```python
from build123d import *

# Parameters (mm, degrees)
BOSS_EXTRUDE1_DEPTH      = 10
BOSS_EXTRUDE2_DEPTH      = 15
BOSS_EXTRUDE2_DEPTH_BACK = 5
SKETCH1_3_R              = 3
SKETCH2_R                = 1.5
CUT_EXTRUDE1_DEPTH       = 39.79576151
BOSS_EXTRUDE3_DEPTH      = 5
BOSS_EXTRUDE3_DEPTH_BACK = 15
SKETCH3_R                = 3


with BuildPart() as part:
    # Sketch1 → Boss-Extrude1 (new body)
    with BuildSketch(Plane.XY):
        with BuildLine():
            Line((-20, 10), (-20, -10))
            Line((-20, -10), (-2.846049894, -15.717983369))
            ThreePointArc((-2.846049894, -15.717983369), (0, -13.666666667), (2.846049894, -15.717983369))
            Line((2.846049894, -15.717983369), (20, -10))
            Line((20, -10), (20, 10))
            Line((20, 10), (-20, 10))
        make_face()
    extrude(amount=BOSS_EXTRUDE1_DEPTH)

    # Sketch1_3 → Boss-Extrude2 (add, two sides: drawn at the far end of the back side and taken through both)
    with BuildSketch(Plane.XY.offset(-BOSS_EXTRUDE2_DEPTH_BACK)):
        with Locations((0, -16.666666667)):
            Circle(SKETCH1_3_R)
    extrude(amount=BOSS_EXTRUDE2_DEPTH + BOSS_EXTRUDE2_DEPTH_BACK)

    # Sketch2 → Cut-Extrude1 (cut, through all)
    with BuildSketch(Plane(origin=(0, 10, 0), x_dir=(1, 0, 0), z_dir=(0, 1, 0))):
        with Locations(Location((-14, -5, 0), (0, 0, 270))):
            Circle(SKETCH2_R)
        with Locations((14, -5)):
            Circle(SKETCH2_R)
    extrude(amount=-CUT_EXTRUDE1_DEPTH, mode=Mode.SUBTRACT)

    # Sketch3 → Boss-Extrude3 (add, two sides: drawn at the far end of the back side and taken through both)
    with BuildSketch(Plane.XY.offset(10).offset(-BOSS_EXTRUDE3_DEPTH_BACK)):
        with Locations((0, 10)):
            Circle(SKETCH3_R)
    extrude(amount=BOSS_EXTRUDE3_DEPTH + BOSS_EXTRUDE3_DEPTH_BACK)


solid = part.part
```
The listing builds one solid part. Answer for the finished solid, in the listing's coordinates (mm). A direction names the side the tool comes from. Round coordinates to 2 decimals unless told otherwise and drop trailing zeros. Loops run counter-clockwise (first coordinate to the right, second up) from the corner with the lowest first, then second, coordinate; pieces in that order, holes last.
Q1. Given pin 1 Ø1.5 at (x, y) = (-5, -3.5) entering from -Z; pin 2 Ø8 at (x, z) = (9, 4.5) entering from +Y; pin 3 Ø6 at (x, y) = (-8.5, 3.5) entering from +Z; pin 4 Ø1.8 at (x, z) = (-14, 5) entering from +Y, each flat-ended and moving along its own axis, determine where each tip first touches the part or whether it passes through.
Q2. Which of the six approach directions +Z, -Z, +X, -X, +Y, -Y give full straight-line access (tool end or side, diameter ignored) to faces 1 (the face through (0, -17, 15)), 2 (the face through (-11, 10, 5))?
Q3. Section D-D, the plane x = 0 is taken. Determine the outline of the cut face in (y, z).
Q4. Find the intervals of material crossed by line 1 (X direction, y = -6.75, z = 5); line 2 (Z direction, x = -14, y = -1.25); line 3 (Z direction, x = -5.5, y = -7), in increasing order.
Q5. For a pull along Y with two mould halves and no side action, classify faces 3 (the face through (-20, 0, 5)), 4 (the face through (0, 13, 5)), 5 (the face through (12, 10, 5)) as released by +Y, released by -Y, zero draft, split by the parting line, or undercut.
Q6. Section B-B, the plane z = 5 is taken. Determine the outline of the cut face in (x, y), then the cut area to 3 significant figures.
Q7. Section C-C, the plane y = -1 is taken. Determine the outline of the cut face in (x, z).
Q8. Section A-A, the plane x = 14 is taken. Determine the outline of the cut face in (y, z), then the cut area to 3 significant figures.
Completed:
1. pin 1: stops at z = 0
1. pin 2: stops at y = 10
1. pin 3: stops at z = 10
1. pin 4: passes through
2. face 1: +Z, +X, -X, +Y, -Y
2. face 2: +Z, -Z, -X, +Y
3. outline: (-19.67, -5) - (-13.67, -5) - (-13.67, 0) - (7, 0) - (7, -5) - (13, -5) - (13, 15) - (7, 15) - (7, 10) - (-13.67, 10) - (-13.67, 15) - (-19.67, 15) - close
4. line 1: x = -20 to -15.5, -12.5 to 12.5, 15.5 to 20
4. line 2: z = 0 to 3.5, 6.5 to 10
4. line 3: z = 0 to 10
5. face 3: zero draft
5. face 4: undercut
5. face 5: released by +Y
6. outline: (-20, -10) - (-15.5, -11.5) - (-15.5, 10) - (-20, 10) - close; (-12.5, -12.5) - (-2.85, -15.72) arc R3 ccw (long way) to (2.85, -15.72) - (12.5, -12.5) - (12.5, 10) - (3, 10) arc R3 ccw to (-3, 10) - (-12.5, 10) - close; (15.5, -11.5) - (20, -10) - (20, 10) - (15.5, 10) - close
6. area: 833 mm2
7. outline: (-20, 0) - (20, 0) - (20, 10) - (-20, 10) - close; hole circle Ø3 at (-14, 5); hole circle Ø3 at (14, 5)
8. outline: (-12, 0) - (10, 0) - (10, 3.5) - (-12, 3.5) - close; (-12, 6.5) - (10, 6.5) - (10, 10) - (-12, 10) - close
8. area: 154 mm2
